```python
from build123d import *

# Parameters (mm, degrees)
SKETCH_1_R           = 10
EXTRUDE_1_DEPTH      = 2
SKETCH_3_R           = 2
SKETCH_3_R_2         = 1.992440636
SKETCH_3_R_3         = 1.836667673
EXTRUDE_2_DEPTH      = 1
EXTRUDE_2_DEPTH_BACK = 1


with BuildPart() as part:
    # Sketch 1 → Extrude 1 (new body)
    with BuildSketch(Plane(origin=(0, 0, 0), x_dir=(1, 0, 0), z_dir=(0, 1, 0))):
        Circle(SKETCH_1_R)
    extrude(amount=EXTRUDE_1_DEPTH)

    # Sketch 3 → Extrude 2 (add, two sides)
    with BuildSketch(Plane.XY) as extrude_2_sk:
        Polygon((9, 2), (-9, 2), (-20, 22), (-20, 32), (-9, 52), (9, 52), (20, 32), (20, 22), align=None)
        with Locations((-7, 47)):
            Circle(SKETCH_3_R, mode=Mode.SUBTRACT)
        with Locations((7, 47)):
            Circle(SKETCH_3_R, mode=Mode.SUBTRACT)
        with Locations((13.7, 27)):
            Circle(SKETCH_3_R_2, mode=Mode.SUBTRACT)
        with Locations((-13.7, 27)):
            Circle(SKETCH_3_R_3, mode=Mode.SUBTRACT)
    extrude(amount=EXTRUDE_2_DEPTH)
    extrude(extrude_2_sk.sketch, amount=-EXTRUDE_2_DEPTH_BACK)


solid = part.part
```
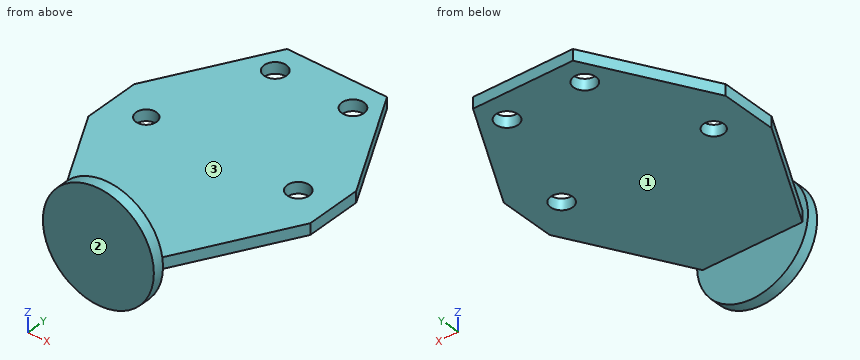
Geometry: final body of the model. Coordinates: model frame, mm. Face numbers are marked on the shaded views. A direction names the side the tool comes from. Coordinates: 2 decimals unless noted, no trailing zeros. Loops run counter-clockwise (first coordinate to the right, second up) from the corner with the lowest first, then second, coordinate; pieces in that order, holes last. Notation, with made-up numbers: M 32,82.25 L 40,82.25 A18 cw 40,100.25 Z; hole C -21.75,-24.75 d5. An arc over 180 degrees is marked long. Put each result on its own line as item: value.
(1) Cut plane D-D on y = 27. Return the cut outline in (x, z), then the cut area to 3 significant figures.
Answer sheet:
outline: M -20,-1 L -15.54,-1 L -15.54,1 L -20,1 Z; M -11.86,-1 L 11.71,-1 L 11.71,1 L -11.86,1 Z; M 15.69,-1 L 20,-1 L 20,1 L 15.69,1 Z
area: 64.7 mm^2
(2) First-contact query: pin 1 (12 mm diameter, centred on x = -2.5, y = 34.5, fed in from +Z); pin 2 (2 mm diameter, centred on y = 8.5, z = 1, fed in from +X) (3 decimals); pin 3 (3 mm diameter, centred on x = 14.5, z = 2, fed in from +Y). Flat tips, straight axial feed; report the tip coordinate or a pass-through.
Answer sheet:
pin 1: stops at z = 1
pin 2: stops at x = 13.125
pin 3: stops at y = 44.03
(3) Access query for the marked faces 1, 2 and 3. Directions: +Z, -Z, +X, -X, +Y, -Y. A direction counts if a zero-diameter tool reaches every point of the face in a straight line with its end or side. Return the directions, or none.
Answer sheet:
face 1: -Z, +X, -X, +Y
face 2: +Z, -Z, +X, -X, -Y
face 3: +Z, +X, -X, +Y
(4) Cut plane C-C on x = 0. Return the cut outline in (y, z).
Answer sheet:
outline: M 0,-10 L 2,-10 L 2,-1 L 52,-1 L 52,1 L 2,1 L 2,10 L 0,10 Z
(5) Material intervals for probe 1 along Z at (x, y) = (-12, 34.5); probe 2 along Y at (x, z) = (6.5, 5.75); probe 3 along Y at (x, z) = (13.7, -0.6), sorted ascending.
Answer sheet:
probe 1: z = -1 to 1
probe 2: y = 0 to 2
probe 3: y = 10.55 to 25.01, 28.99 to 43.45
(6) Cut plane B-B on x = -14.5. Return the cut outline in (y, z), then the cut area to 3 significant figures.
Answer sheet:
outline: M 12,-1 L 25.35,-1 L 25.35,1 L 12,1 Z; M 28.65,-1 L 42,-1 L 42,1 L 28.65,1 Z
area: 53.4 mm^2
(7) Cut plane A-A on y = 47. Return the cut outline in (x, z), then the cut area to 3 significant figures.
Answer sheet:
outline: M -11.75,-1 L -9,-1 L -9,1 L -11.75,1 Z; M -5,-1 L 5,-1 L 5,1 L -5,1 Z; M 9,-1 L 11.75,-1 L 11.75,1 L 9,1 Z
area: 31.0 mm^2
